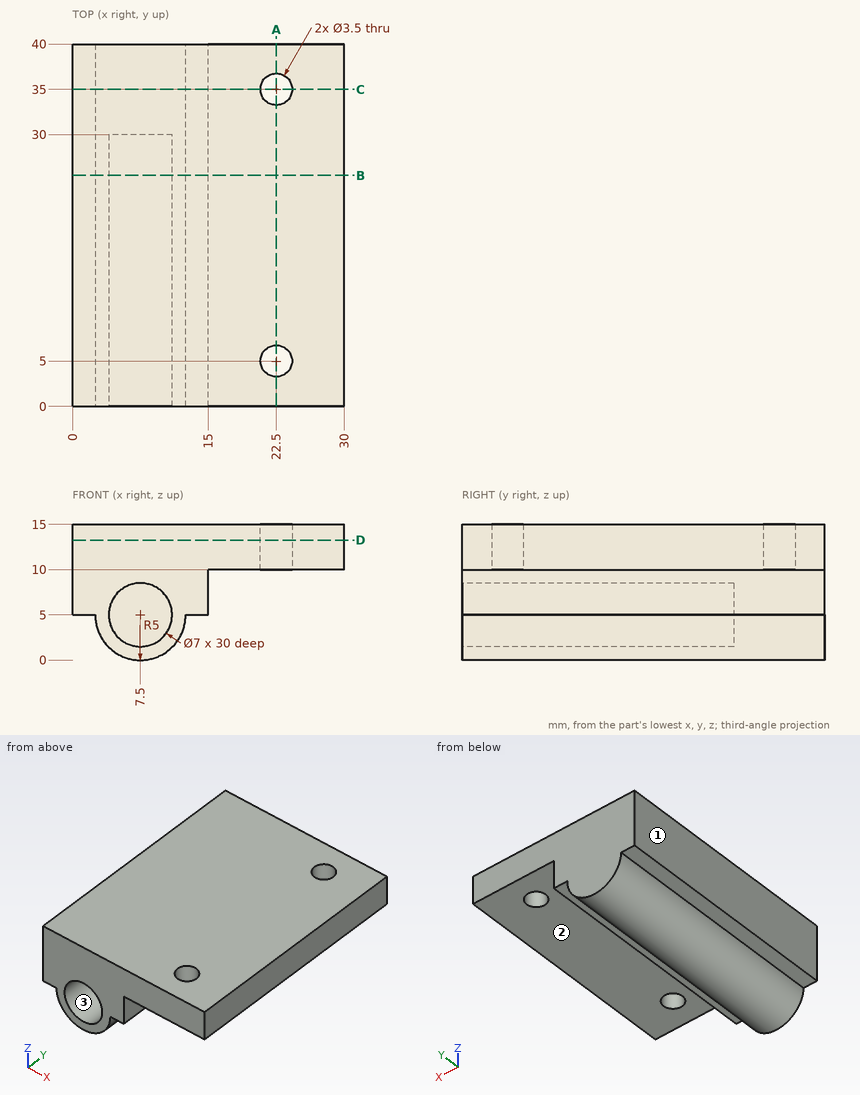
Geometry: see drawing. Coordinates: mm, zero at the bounding-box minimum. Give positions to 0.01 mm unless a question says otherwise; leave off trailing zeros. Loops run counter-clockwise (first coordinate to the right, second up) from the corner with the lowest first, then second, coordinate; pieces in that order, holes last. Notation, with made-up numbers: M 16,76.5 L 33,76.5 A29 ccw 33,111.5 Z; hole C -2.75,87.25 d11. An arc over 180 degrees is marked long. Answer as CSV lines item,"result". Start each with the question number.
1. Section D-D on z = 13.25. Return loops of the section in (x, y), plus the area to 3 significant figures.
2. Pin query (flat end, axial travel): P1, Ø4, axis at y = 24, z = 7, coming from the +X side; P2, Ø3, axis at x = 22.5, y = 35, coming from the +Z side; P3, Ø5, axis at x = 23, y = 4, coming from the -Z side; P4, Ø0.8, axis at x = 1.5, y = 15.5, coming from the -Z side. Return the tip coordinate at first contact, or that it passes through.
3. Section B-B on y = 25.5. Return loops of the section in (x, z), plus the area to 3 significant figures.
4. Pull-direction query (X, two-part tool) for the marked faces 1, 2 and 3; classes: released by +X, released by -X, zero draft, split by the parting line, or undercut.
5. Line query: L1, parallel to Y at x = 22.5, z = 12.4; L2, parallel to Z at x = 7.5, y = 19; L3, parallel to Z at x = 23, y = 30. Output: solid intervals per line, ascending.
6. Section A-A on x = 22.5. Return loops of the section in (y, z).
7. Section C-C on y = 35. Return loops of the section in (x, z), plus the area to 3 significant figures.
Computed values:
1,outline,"M 0,0 L 30,0 L 30,40 L 0,40 Z; hole C 22.5,5 d3.5; hole C 22.5,35 d3.5"
1,area,"1,180 mm²"
2,P1,"stops at x = 15"
2,P2,"passes through"
2,P3,"stops at z = 10"
2,P4,"stops at z = 5"
3,outline,"M 0,5 L 2.5,5 A5 ccw 12.5,5 L 15,5 L 15,10 L 30,10 L 30,15 L 0,15 Z; hole C 7.5,5 d7"
3,area,"226 mm²"
4,face 1,"released by -X"
4,face 2,"zero draft"
4,face 3,"undercut"
5,L1,"y = 0 to 3.25, 6.75 to 33.25, 36.75 to 40"
5,L2,"z = 0 to 1.5, 8.5 to 15"
5,L3,"z = 10 to 15"
6,outline,"M 0,10 L 3.25,10 L 3.25,15 L 0,15 Z; M 6.75,10 L 33.25,10 L 33.25,15 L 6.75,15 Z; M 36.75,10 L 40,10 L 40,15 L 36.75,15 Z"
7,outline,"M 0,5 L 2.5,5 A5 ccw 12.5,5 L 15,5 L 15,10 L 20.75,10 L 20.75,15 L 0,15 Z; M 24.25,10 L 30,10 L 30,15 L 24.25,15 Z"
7,area,"247 mm²"
